Geometry: final body of the model. Coordinates: model frame, mm. Face numbers are marked on the shaded views. Give positions to 0.01 mm unless a question says otherwise; leave off trailing zeros. Order: outer loops, then holes, each group sorted by start corner. A loop starts at its lowest first (then second) coordinate and runs counter-clockwise, first axis right, second up. Notation, with made-up numbers: M 33,-35.75 L 81,-35.75 A11 cw 81,-14.75 Z; hole C 44,79.25 d1. An arc over 180 degrees is marked long. One line per item, written item: value. Start each with the question number.
```python
from build123d import *

# Parameters (mm, degrees)
F0_R     = 0.5
F1_DEPTH = 9
F2_W     = 3.75
F2_H     = 2
F3_DEPTH = 1.501


with BuildPart() as f1:
    # F0 (on Right) → F1 (new body)
    with BuildSketch(Plane.YZ):
        with BuildLine():
            ThreePointArc((0, 1.5), (-0.75, 0.75), (0, 0))
            Line((0, 0), (20, 0))
            ThreePointArc((20, 0), (20.75, 0.75), (20, 1.5))
            Line((20, 1.5), (0, 1.5))
        make_face()
        with Locations((0, 0.75)):
            Circle(F0_R, mode=Mode.SUBTRACT)
        with Locations((20, 0.75)):
            Circle(F0_R, mode=Mode.SUBTRACT)
    extrude(amount=F1_DEPTH)

    # F2 (on Top) → F3 (cut, through all)
    with BuildSketch(Plane.XY):
        with Locations((4.5, 19.75)):
            Rectangle(F2_W, F2_H)
    extrude(amount=F3_DEPTH, mode=Mode.SUBTRACT)


solid = f1.part
```
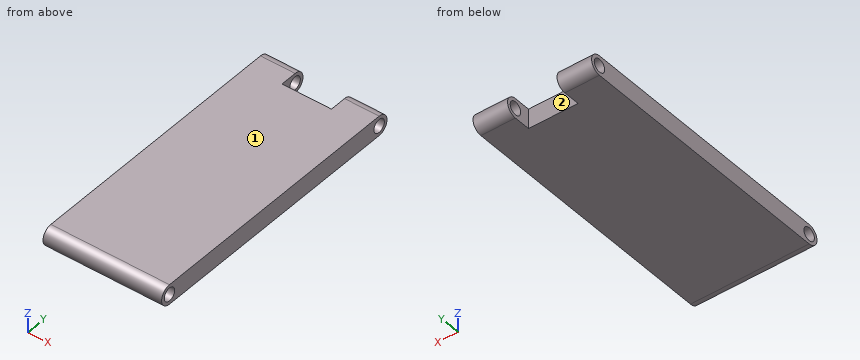
Q1. Contact query for a flat-ended pin moving along its axis: pin 1 (0.8 mm diameter, centred on x = 4.5, z = 0.5, fed in from +Y). Output: stop coordinate, or through.
Q2. Section query C-C on x = 1. Return loops of the section in (y, z).
Q3. Section query B-B on z = 0.75. Return loops of the section in (x, y) (3 decimals), and give its area (3 significant figures).
Q4. Ray query, line 1 along Y through (x, z) = (1.5, 0.8); line 2 along Z through (x, y) = (7.4, 20); line 3 along X through (y, z) = (19.5, 0.35) (3 decimals). Return the intervals inside material, ascending. Write a range as [from, to].
Q5. Section query A-A on x = 5. Return loops of the section in (y, z), and give its area (3 significant figures).
Q6. Mould query, pull axis X, two halves, no side actions, for the marked faces 1 and 2. Classes: +X half, -X half, draft (parallel to the pull), parting line (faces both ways), or undercut.
Results below:
1. pin 1: y = 18.75
2. outline: M 0,0 L 20,0 A0.75 ccw 20,1.5 L 0,1.5 A0.75 ccw Z; hole C 0,0.75 d1; hole C 20,0.75 d1
3. outline: M 0,-0.75 L 9,-0.75 L 9,-0.5 L 0,-0.5 Z; M 0,0.5 L 9,0.5 L 9,19.5 L 6.375,19.5 L 6.375,18.75 L 2.625,18.75 L 2.625,19.5 L 0,19.5 Z; M 0,20.5 L 2.625,20.5 L 2.625,20.75 L 0,20.75 Z; M 6.375,20.5 L 9,20.5 L 9,20.75 L 6.375,20.75 Z
3. area: 172 mm2
4. line 1: [-0.75, -0.5], [0.5, 19.5], [20.5, 20.75]
4. line 2: [0, 0.25], [1.25, 1.5]
4. line 3: [0, 2.625], [6.375, 9]
5. outline: M 0,0 L 18.75,0 L 18.75,1.5 L 0,1.5 A0.75 ccw Z; hole C 0,0.75 d1
5. area: 28.2 mm2
6. face 1: draft
6. face 2: undercut
